```python
from build123d import *

# Parameters (mm, degrees)
F0_R     = 7.625
F1_DEPTH = 34.925
F2_DEPTH = 9.525
F3_DEPTH = 22.225
F5_DEPTH = 7


with BuildPart() as f1:
    # F0 (on Top) → F1 (new body)
    with BuildSketch(Plane.XY):
        Circle(F0_R)
        with BuildLine():
            ThreePointArc((5.0990195136, 2.375), (5.4919308883, 1.2162730442), (5.625, 0))
            ThreePointArc((5.625, 0), (-1.2162730442, -5.4919308883), (-5.0990195136, 2.375))
            ThreePointArc((-5.0990195136, 2.375), (0, 5.625), (5.0990195136, 2.375))
        make_face(mode=Mode.SUBTRACT)
        with BuildLine():
            ThreePointArc((-5.0990195136, 2.375), (-1.2162730442, -5.4919308883), (5.625, 0))
            ThreePointArc((5.625, 0), (5.4919308883, 1.2162730442), (5.0990195136, 2.375))
            Line((5.0990195136, 2.375), (-5.0990195136, 2.375))
        make_face()
        with BuildLine():
            Line((-5.0990195136, 2.375), (5.0990195136, 2.375))
            ThreePointArc((5.0990195136, 2.375), (0, 5.625), (-5.0990195136, 2.375))
        make_face()
    extrude(amount=F1_DEPTH)

    # F0 (on Top) → F2 (cut)
    with BuildSketch(Plane.XY):
        with BuildLine():
            ThreePointArc((-5.0990195136, 2.375), (-1.2162730442, -5.4919308883), (5.625, 0))
            ThreePointArc((5.625, 0), (5.4919308883, 1.2162730442), (5.0990195136, 2.375))
            Line((5.0990195136, 2.375), (-5.0990195136, 2.375))
        make_face()
        with BuildLine():
            Line((-5.0990195136, 2.375), (5.0990195136, 2.375))
            ThreePointArc((5.0990195136, 2.375), (0, 5.625), (-5.0990195136, 2.375))
        make_face()
    extrude(amount=F2_DEPTH, mode=Mode.SUBTRACT)

    # F0 (on Top) → F3 (cut)
    with BuildSketch(Plane.XY):
        with BuildLine():
            ThreePointArc((-5.0990195136, 2.375), (-1.2162730442, -5.4919308883), (5.625, 0))
            ThreePointArc((5.625, 0), (5.4919308883, 1.2162730442), (5.0990195136, 2.375))
            Line((5.0990195136, 2.375), (-5.0990195136, 2.375))
        make_face()
    extrude(amount=F3_DEPTH, mode=Mode.SUBTRACT)

    # F4 (on face) → F5 (join)
    with BuildSketch(Plane.XY.offset(34.925)):
        with BuildLine():
            Line((2.5, -7.2035147671), (2.5, 7.2035147671))
            ThreePointArc((2.5, 7.2035147671), (0, 7.625), (-2.5, 7.2035147671))
            Line((-2.5, 7.2035147671), (-2.5, -7.2035147671))
            ThreePointArc((-2.5, -7.2035147671), (0, -7.625), (2.5, -7.2035147671))
        make_face()
    extrude(amount=F5_DEPTH)


solid = f1.part
```
Read the model definition and answer for the solid it produces. Units are mm, in the model's axes. A direction names the side the tool comes from. Give positions to 0.01 mm unless a question says otherwise; leave off trailing zeros. Loops run counter-clockwise (first coordinate to the right, second up) from the corner with the lowest first, then second, coordinate; pieces in that order, holes last.
Item 1: The part is cut by section C-C (y = 0). Write down the section's boundary in (x, z) (3 decimals).
Item 2: Each of these flat-tipped pins is pushed along its axis until it touches: pin 1 Ø4 at (x, y) = (6.5, 2.5) entering from +Z (3 decimals); pin 2 Ø2 at (x, z) = (-2.5, 19.5) entering from -Y; pin 3 Ø2.5 at (x, y) = (2, 3.5) entering from -Z (3 decimals). Where does it stop, or does it pass through?
Item 3: The mould has two halves that part along X. Classify faces 1 (the flat face through (-1, -6, 0)), 2 (the flat face through (0, 2.375, 16)), 3 (the flat face through (2.5, 0, 38)): released by +X, released by -X, zero draft, split by the parting line, or undercut.
Item 4: The part is cut by section D-D (z = 30.5). Write down the section's boundary in (x, y) (3 decimals), and give its area (3 significant figures).
Item 5: The part is cut by section B-B (z = 21). Write down the section's boundary in (x, y) (3 decimals), and give its area (3 significant figures).
Item 6: Find the intervals of material crossed by line 1 along Y through (x, z) = (0, 7) (3 decimals); line 2 along Z through (x, y) = (-3, 0.25) (3 decimals); line 3 along Z through (x, y) = (3.25, 4.25) (3 decimals), in increasing order.
Item 7: The part is cut by section A-A (x = 0). Write down the section's boundary in (y, z) (3 decimals).
Item 8: For faces 4 (the flat face through (4, 0, 34.925)), 5 (the flat face through (-5, 0, 34.925)), 6 (the cylindrical face through (-1.22, -5.49, 10.96)), 7 (the flat face through (0, 0, 41.925)), determine the directions among +Z, -Z, +X, -X, +Y, -Y from which every point of the face is accessible in a straight line to the end or side of a thin tool.
Taken from the geometry:
1. outline: (-7.625, 0) - (-5.625, 0) - (-5.625, 22.225) - (5.625, 22.225) - (5.625, 0) - (7.625, 0) - (7.625, 34.925) - (2.5, 34.925) - (2.5, 41.925) - (-2.5, 41.925) - (-2.5, 34.925) - (-7.625, 34.925) - close
2. pin 1: stops at z = 34.925
2. pin 2: stops at y = -7.48
2. pin 3: stops at z = 9.525
3. face 1: zero draft
3. face 2: undercut
3. face 3: released by +X
4. outline: circle Ø15.25 at (0, 0)
4. area: 183 mm2
5. outline: circle Ø15.25 at (0, 0); hole (-5.099, 2.375) arc R5.625 ccw (long way) to (5.099, 2.375) - close
5. area: 107 mm2
6. line 1: y = -7.625 to -5.625, 5.625 to 7.625
6. line 2: z = 22.225 to 34.925
6. line 3: z = 9.525 to 34.925
7. outline: (-7.625, 0) - (-5.625, 0) - (-5.625, 22.225) - (2.375, 22.225) - (2.375, 9.525) - (5.625, 9.525) - (5.625, 0) - (7.625, 0) - (7.625, 41.925) - (-7.625, 41.925) - close
8. face 4: +Z, +X, +Y, -Y
8. face 5: +Z, -X, +Y, -Y
8. face 6: -Z
8. face 7: +Z, +X, -X, +Y, -Y
